Study the drawing (mm; zero at the part's minimum x, y, z) and answer. Coordinates: 2 decimals unless noted, no trailing zeros. Loops run counter-clockwise (first coordinate to the right, second up) from the corner with the lowest first, then second, coordinate; pieces in that order, holes last. Notation, with made-up numbers: (45.5, 82) - (74.5, 82) arc R23 cw to (74.5, 102) - close; hole circle Ø11 at (57, 18). An arc over 180 degrees is marked (long way). Put each result on its own line as item: value.
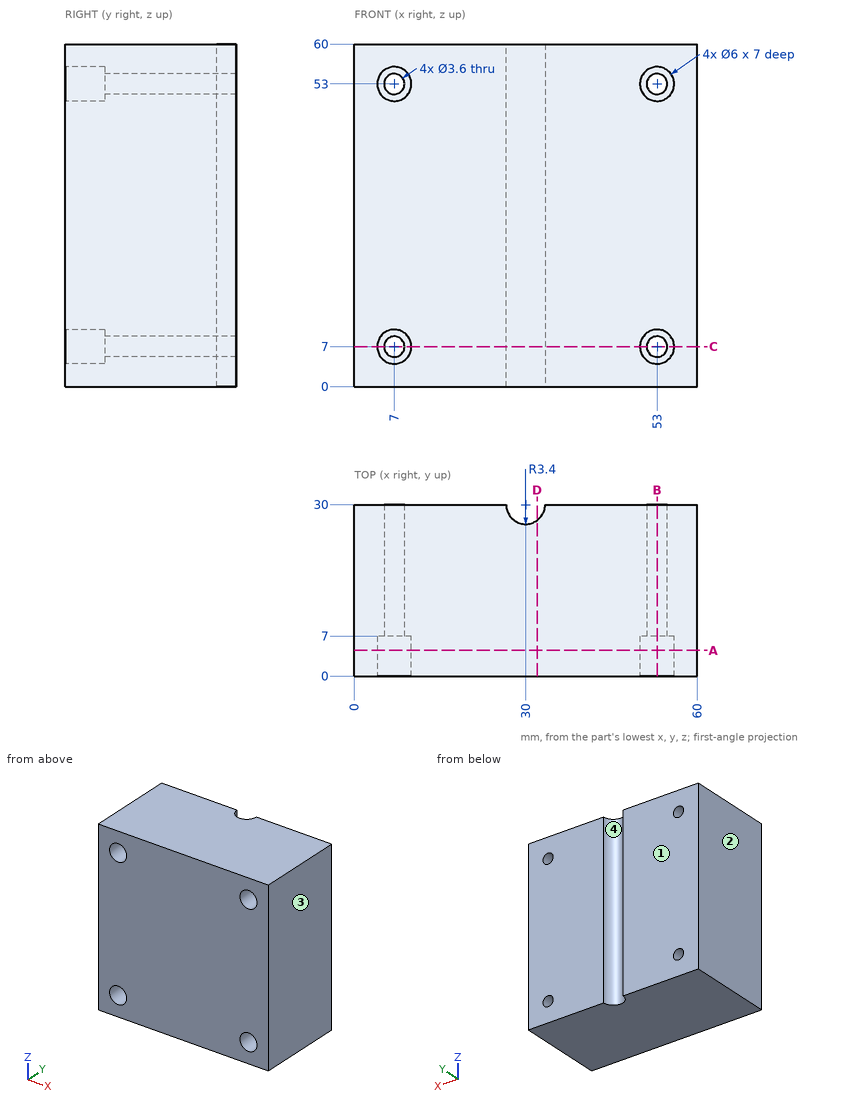
1) The part is cut by section D-D (x = 32). Give the vertices of the cut face in (y, z), and give its area (3 significant figures).
Found:
outline: (0, 0) - (27.25, 0) - (27.25, 60) - (0, 60) - close
area: 1,640 mm^2
2) For a pull along X with two mould halves and no side action, classify the marked faces 1, 2, 3 and 4 as pulls with the +X half, pulls with the -X half, needs draft (parallel to the pull), parting line crosses it, or undercut.
Found:
face 1: needs draft
face 2: pulls with the -X half
face 3: pulls with the +X half
face 4: undercut
3) The part is cut by section B-B (x = 53). Give the vertices of the cut face in (y, z).
Found:
outline: (0, 0) - (30, 0) - (30, 5.2) - (7, 5.2) - (7, 4) - (0, 4) - close; (0, 10) - (7, 10) - (7, 8.8) - (30, 8.8) - (30, 51.2) - (7, 51.2) - (7, 50) - (0, 50) - close; (0, 56) - (7, 56) - (7, 54.8) - (30, 54.8) - (30, 60) - (0, 60) - close
4) Straight lines are drawn through the part: L1, parallel to Z at x = 7, y = 20.5; L2, parallel to Z at x = 53, y = 5; L3, parallel to X at y = 27, z = 54.5. For each, find the intervals that lie inside material, in ascending order. Write a range as [from, to].
Found:
L1: z = [0, 5.2], [8.8, 51.2], [54.8, 60]
L2: z = [0, 4], [10, 50], [56, 60]
L3: x = [0, 6.01], [7.99, 28.4], [31.6, 52.01], [53.99, 60]
5) Each of these flat-tipped pins is pushed along its axis until it touches: pin 1 (1.8 mm diameter, centred on x = 53, z = 52, fed in from -Y); pin 2 (3.5 mm diameter, centred on x = 53, z = 53, fed in from +Y). Where does it stop, or does it pass through?
Found:
pin 1: stops at y = 7
pin 2: passes through
6) The part is cut by section C-C (z = 7). Give the vertices of the cut face in (x, y), and give its area (3 significant figures).
Found:
outline: (0, 0) - (4, 0) - (4, 7) - (5.2, 7) - (5.2, 30) - (0, 30) - close; (8.8, 7) - (10, 7) - (10, 0) - (50, 0) - (50, 7) - (51.2, 7) - (51.2, 30) - (33.4, 30) arc R3.4 cw to (26.6, 30) - (8.8, 30) - close; (54.8, 7) - (56, 7) - (56, 0) - (60, 0) - (60, 30) - (54.8, 30) - close
area: 1,530 mm^2
7) The part is cut by section A-A (y = 4.5). Give the vertices of the cut face in (x, z).
Found:
outline: (0, 0) - (60, 0) - (60, 60) - (0, 60) - close; hole circle Ø6 at (7, 7); hole circle Ø6 at (7, 53); hole circle Ø6 at (53, 7); hole circle Ø6 at (53, 53)
